The listing builds one solid part. Answer for the finished solid, in the listing's coordinates (mm). A direction names the side the tool comes from. Give positions to 0.01 mm unless a question says otherwise; leave off trailing zeros. Write each loop counter-clockwise with the first axis right and the second up, starting at its lowest first coordinate (ties: lowest second). Pieces come first, ordered by that corner, then holes. Notation, with made-up numbers: (-21, 6.25) - (12, 6.25) arc R15 cw to (12, 33.25) - close; hole circle Ø10 at (72.25, 77). An arc over 180 degrees is marked (long way). Write each question's results on one line, items separated by ' | '. Start each with the question number.
Q1. Find the intervals of material crossed by probe 1 along X at (y, z) = (9, 0); probe 2 along Z at (x, y) = (2.25, -0.5); probe 3 along Z at (x, y) = (1.5, 11.5), in increasing order.
Q2. Section C-C (z = 1) is taken. Determine the outline of the cut face in (x, y), plus the area to 3 significant figures.
Q3. For a pull along Z with two mould halves and no side action, classify faces 1 (the face through (1.5, -14.6, 1.2)), 2 (the face through (7.93, 6.654, -3.461)), 3 (the face through (13, 3, 6)) as pulls with the +Z half, pulls with the -Z half, needs draft (parallel to the pull), parting line crosses it, or undercut.
Q4. Section B-B (y = 13) is taken. Determine the outline of the cut face in (x, z), plus the area to 3 significant figures.
Q5. Flat-ended cylindrical pins translate along their axes: pin 1 Ø2.5 at (y, z) = (13, 0) entering from -X; pin 2 Ø3 at (x, z) = (1.5, -6) entering from +Y; pin 3 Ø1.5 at (x, y) = (10, -1) entering from -Z; pin 4 Ø2 at (x, y) = (10, 7) entering from -Z. Find the tip coordinate at first contact, or state that the pin passes through.
Q6. For faces 4 (the face through (3, 6.89, -3.33)), 5 (the face through (1.5, 11.4, 1.2)), determine the directions among +Z, -Z, +X, -X, +Y, -Y from which every point of the face is accessible in a straight line to the end or side of a thin tool.
Q7. Section A-A (x = 7.25) is taken. Determine the outline of the cut face in (y, z), plus the area to 3 significant figures.
Autodesk Inventor part; units mm, degrees
ref_plane "Work Plane1" through (0, 0, 0) normal (0, 0.7071, -0.7071) x (-1, 0, 0)
ref_plane "YZ Plane" through (0, 0, 0) normal (1, 0, 0) x (0, 1, 0)
sketch "Sketch1" plane through (0, 0, 0) normal (1, 0, 0) x (0, 1, 0)
  circle A0 centre (0, 0) radius 16
  circle A1 centre (0, 13) radius 2
  circle A2 centre (0, -13) radius 2
  circle A3 centre (-13, 0) radius 2
  circle A4 centre (13, 0) radius 2
  circle A5 centre (0, -13) radius 2
  circle A6 centre (0, 13) radius 2
  circle A7 centre (13, 0) radius 2
  circle A8 centre (-13, 0) radius 2
  circle A9 centre (0, 0) radius 6.35
  line L0 (0, -22.4) -> (0, 22.4)
  dimension "d0" = 32
  dimension "d1" = 4
  dimension "d2" = 26
  dimension "d3" = 13
  dimension "d6" = 360
  dimension "d8" = 12.7
extrude "Extrusion1" add sketch "Sketch1" along normal blind 3 contours A0 L0 A2 A9 A1 | L0 A1 A9 A2 A0
sketch "Sketch2" plane through (3, 0, 0) normal (1, 0, 0) x (0, 0, -1)
  circle A0 centre (0, 0) radius 16
  circle A1 centre (13, 0) radius 2
  circle A2 centre (0, 0) radius 6.35
  circle A3 centre (0, -13) radius 2
  circle A4 centre (-13, 0) radius 2
  circle A5 centre (0, 13) radius 2
  circle A6 centre (0, 0) radius 7.5
  dimension "d11" = 15
extrude "Extrusion2" add sketch "Sketch2" along normal blind 10 contours A6
ref_plane "Work Plane1" through (0, 0, 0) normal (0, 0.7071, -0.7071) x (-1, 0, 0)
sketch "Sketch5" plane through (0, 0, 0) normal (0, 0.7071, -0.7071) x (-1, 0, 0)
  circle A0 centre (-8, 0) radius 2
  line L0 (-13, 7.5) -> (-13, -7.5)
  line L1 (-3, -7.5) -> (-3, 7.5)
  point P0 (0, 0)
  point P1 (-13, 0)
  dimension "d14" = 4
  dimension "d15" = 5
extrude "Extrusion3" cut sketch "Sketch5" along normal through all both and the other way through all
properties part number "HipCoupler"
Answers below:
1) probe 1: x = 0 to 3 | probe 2: z = -15.99 to -14.94, -11.06 to -6.33, 6.33 to 11.06, 14.94 to 15.99 | probe 3: z = -11.12 to -1.32, 1.32 to 11.12
2) outline: (0, -15.97) - (3, -15.97) - (3, -14.73) - (0, -14.73) - close; (0, -11.27) - (3, -11.27) - (3, -7.43) - (13, -7.43) - (13, -6.27) - (0, -6.27) - close; (0, 6.27) - (13, 6.27) - (13, 7.43) - (3, 7.43) - (3, 11.27) - (0, 11.27) - close; (0, 14.73) - (3, 14.73) - (3, 15.97) - (0, 15.97) - close | area: 60.6 mm2
3) face 1: undercut | face 2: parting line crosses it | face 3: needs draft
4) outline: (0, -9.33) - (3, -9.33) - (3, -2) - (0, -2) - close; (0, 2) - (3, 2) - (3, 9.33) - (0, 9.33) - close | area: 44.0 mm2
5) pin 1: passes through | pin 2: stops at y = 15.35 | pin 3: stops at z = -7.5 | pin 4: stops at z = -4.5
6) face 4: +X | face 5: +X, -X
7) outline: (-6.45, 3.83) arc R7.5 ccw to (3.83, -6.45) - (2.98, -5.61) arc R6.35 cw to (-5.61, 2.98) - close; (-3.83, 6.45) - (-2.98, 5.61) arc R6.35 cw to (5.61, -2.98) - (6.45, -3.83) arc R7.5 ccw to start | area: 41.4 mm2
